The listing builds one solid part. Answer for the finished solid, in the listing's coordinates (mm). A direction names the side the tool comes from. Round coordinates to 2 decimals unless told otherwise and drop trailing zeros. Write each loop counter-clockwise with the first axis right and the second up, starting at its lowest first coordinate (ties: lowest second). Pieces come first, ordered by that corner, then holes. Notation, with made-up numbers: M -12,-28 L 3,-28 A20 cw 3,-22 Z; hole C 8,-18 d2. An arc over 180 degrees is marked long. One line per item, written item: value. Start each with the question number.
(1) Consider probe 1 along Y at (x, z) = (9.25, 0); probe 2 along Z at (x, y) = (8.75, -1). Determine where each line is inside the solid, lowest interval first.
(2) For faces 1 (the cylindrical face through (8.99, -1.08, 4.88)), 2 (the cylindrical face through (6.06, -0.75, -5.7)), 3 (the cylindrical face through (-9.01, -1.08, 4.88)), determine the directions among +Z, -Z, +X, -X, +Y, -Y from which every point of the face is accessible in a straight line to the end or side of a thin tool.
(3) Section B-B (y = 5.25) is taken. Determine the outline of the cut face in (x, z), plus the area to 3 significant figures.
(4) Given P1, Ø2, axis at x = 3.5, y = -3.5, coming from the -Z side; P2, Ø3.5, axis at y = -0.5, z = 0.5, coming from the +X side; P3, Ø2, axis at x = -3, y = 1.5, coming from the -Z side; P4, Ø4, axis at x = 5, z = -4, coming from the -Y side, each flat-ended and moving along its own axis, determine where each tip first touches the part or whether it passes through.
(5) Section A-A (x = -7.5) is taken. Determine the outline of the cut face in (y, z), plus the area to 3 significant figures.
(6) For a pull along X with two mould halves and no side action, classify faces 4 (the cylindrical face through (-8, -6, 0)), 5 (the flat face through (-9.5, -1, -3)), 6 (the cylindrical face through (-6.04, -0.75, -5.7)) as released by +X, released by -X, zero draft, split by the parting line, or undercut.
(7) Section D-D (x = 6.25) is taken. Determine the outline of the cut face in (y, z).
```python
from build123d import *


with BuildPart() as part:
    # Esboço1 → Revolução1 (revolve)
    with BuildSketch(Plane.XY):
        Polygon((-9.5, 6), (-6.6, 6), (-6.6, 5.75), (-5.5, 5.75), (-5.5, 6), (5.5, 6), (5.5, 5.75), (6.6, 5.75), (6.6, 6), (9.5, 6), (9.5, 5), (8.5, 5), (8.5, 4), (9.5, 4), (9.5, 3), (-9.5, 3), (-9.5, 4), (-8.5, 4), (-8.5, 5), (-9.5, 5), align=None)
    revolve(axis=Axis((0, 0, 0), (-1, 0, 0)))


solid = part.part
```
Recorded:
1. probe 1: y = -6 to -5, -4 to -3, 3 to 4, 5 to 6
1. probe 2: z = -5.92 to -4.9, -3.87 to -2.83, 2.83 to 3.87, 4.9 to 5.92
2. face 1: +X
2. face 2: none
2. face 3: -X
3. outline: M -9.5,-2.9 L -6.6,-2.9 L -6.6,-2.35 L -5.5,-2.35 L -5.5,-2.9 L 5.5,-2.9 L 5.5,-2.35 L 6.6,-2.35 L 6.6,-2.9 L 9.5,-2.9 L 9.5,2.9 L 6.6,2.9 L 6.6,2.35 L 5.5,2.35 L 5.5,2.9 L -5.5,2.9 L -5.5,2.35 L -6.6,2.35 L -6.6,2.9 L -9.5,2.9 Z
3. area: 108 mm2
4. P1: stops at z = -5.45
4. P2: passes through
4. P3: stops at z = -5.98
4. P4: stops at y = -5.66
5. outline: C 0,0 d12; hole C 0,0 d6
5. area: 84.8 mm2
6. face 4: zero draft
6. face 5: released by -X
6. face 6: undercut
7. outline: C 0,0 d11.5; hole C 0,0 d6
